Here's the drawing with two shaded views (mm, measured from the low corner). I have some questions. Coordinates: 2 decimals unless noted, no trailing zeros. Order: outer loops, then holes, each group sorted by start corner. A loop starts at its lowest first (then second) coordinate and runs counter-clockwise, first axis right, second up. Notation, with made-up numbers: (73, 65) -> (113, 65) arc R24 ccw to (113, 97) -> close; hole circle Ø4 at (-15.75, 2). An arc over 180 degrees is marked (long way). Write item = value, one per line.
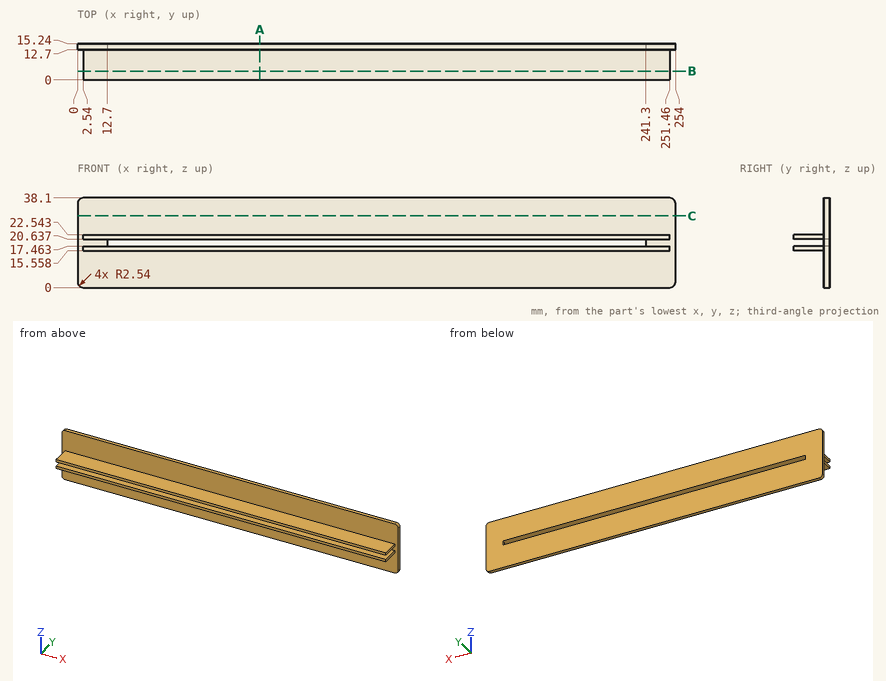
Item 1: I want a section at C-C, the plane z = 30.5. Please give me the cut outline in (x, y).
A:
outline = (0, 12.7) -> (254, 12.7) -> (254, 15.24) -> (0, 15.24) -> close
Item 2: I'm going to push flat-ended pins straight in: P1, Ø5, axis at x = 140.5, z = 28.5, coming from the -Y side; P2, Ø1.5, axis at x = 197, y = 11.5, coming from the -Z side; P3, Ø2, axis at y = 4, z = 22, coming from the -X side. Where does each tip first touch, or does it pass through?
A:
P1 = 12.7
P2 = 15.56
P3 = 2.54
Item 3: I want a section at A-A, the plane x = 77.5. Please give me the cut outline in (y, z), plus the area to 3 significant figures.
A:
outline = (0, 15.56) -> (12.7, 15.56) -> (12.7, 0) -> (15.24, 0) -> (15.24, 17.46) -> (0, 17.46) -> close; (0, 20.64) -> (15.24, 20.64) -> (15.24, 38.1) -> (12.7, 38.1) -> (12.7, 22.54) -> (0, 22.54) -> close
area = 137 mm2
Item 4: I want a section at B-B, the plane y = 3.75. Please give me the cut outline in (x, z).
A:
outline = (2.54, 15.56) -> (251.46, 15.56) -> (251.46, 17.46) -> (2.54, 17.46) -> close; (2.54, 20.64) -> (251.46, 20.64) -> (251.46, 22.54) -> (2.54, 22.54) -> close
Item 5: If I drill on probe 1 along Z at (x, y) = (14, 13); probe 2 along Z at (x, y) = (19, 6.5); probe 3 along Y at (x, z) = (126.5, 5.5), over which ranges is the centre line in solid material (lowest first)?
A:
probe_1 = 0 to 17.46, 20.64 to 38.1
probe_2 = 15.56 to 17.46, 20.64 to 22.54
probe_3 = 12.7 to 15.24
